```python
from build123d import *
from build123d.topology import SkipClean

# Parameters (mm, degrees)
SKETCH_1_W          = 63
SKETCH_1_H          = 15
SKETCH_1_R          = 1.5
SKETCH_1_R_2        = 1.1
SKETCH_1_R_3        = 2.6
EXTRUDE_1_DEPTH     = 2
SKETCH_2_R          = 1.4
EXTRUDE_2_DEPTH     = 2
SKETCH_3_R          = 3
CUT_EXTRUDE_1_DEPTH = 1.5
SKETCH_4_W          = 46
SKETCH_4_H          = 1.5
EXTRUDE_3_DEPTH     = 5
SKETCH_2_3_R        = 0.95
CUT_EXTRUDE_2_DEPTH = 1.5
CUT_EXTRUDE_3_DEPTH = 0.25
SKETCH_1_7_W        = 15
SKETCH_1_7_H        = 15
SKETCH_1_7_R        = 1.5
SKETCH_1_7_R_2      = 1.1
EXTRUDE_4_DEPTH     = 4
SKETCH_1_8_R        = 6
SKETCH_1_8_R_2      = 1.5
SKETCH_1_8_R_3      = 1.1
CUT_EXTRUDE_4_DEPTH = 2
CUT_EXTRUDE_5_DEPTH = 15
EXTRUDE_START       = 3
SKETCH_8_R          = 5.5
SKETCH_8_R_2        = 2.6
EXTRUDE_11_DEPTH    = 3
CUT_EXTRUDE_6_DEPTH = 3.5
CUT_EXTRUDE_7_DEPTH = 3
SKETCH_8_2_R        = 5.5
SKETCH_8_2_R_2      = 2.6
EXTRUDE_12_DEPTH    = 4


with BuildPart() as part:
    # 草图1 → 凸台-拉伸1 (new body)
    with BuildSketch(Plane(origin=(0, 0, 0), x_dir=(1, 0, 0), z_dir=(0, 1, 0))):
        Rectangle(SKETCH_1_W, SKETCH_1_H)
        with Locations(Location((-8.5, 0, 0), (0, 0, 270))):
            Circle(SKETCH_1_R, mode=Mode.SUBTRACT)
        with Locations(Location((-4.169872981, 2.5, 0), (0, 0, 270))):
            Circle(SKETCH_1_R_2, mode=Mode.SUBTRACT)
        with Locations(Location((-12.830127019, -2.5, 0), (0, 0, 270))):
            Circle(SKETCH_1_R_2, mode=Mode.SUBTRACT)
        with Locations(Location((8, 0, 0), (0, 0, 270))):
            Circle(SKETCH_1_R_3, mode=Mode.SUBTRACT)
        with Locations(Location((24, 0, 0), (0, 0, 270))):
            Circle(SKETCH_1_R, mode=Mode.SUBTRACT)
        with Locations(Location((27.5, 0, 0), (0, 0, 270))):
            Circle(SKETCH_1_R_2, mode=Mode.SUBTRACT)
        with Locations(Location((24, -3.5, 0), (0, 0, 270))):
            Circle(SKETCH_1_R_2, mode=Mode.SUBTRACT)
        with Locations(Location((20.5, 0, 0), (0, 0, 270))):
            Circle(SKETCH_1_R_2, mode=Mode.SUBTRACT)
        with Locations(Location((24, 3.5, 0), (0, 0, 270))):
            Circle(SKETCH_1_R_2, mode=Mode.SUBTRACT)
    extrude(amount=EXTRUDE_1_DEPTH)

    # 草图2 → 凸台-拉伸2 (add)
    with BuildSketch(Plane.XY.offset(7.5)):
        with Locations(Location((-23.5, 0.6, 0), (0, 0, 205.376933525))):
            Circle(SKETCH_2_R)
        with Locations(Location((-8.5, 0.6, 0), (0, 0, 205.376933525))):
            Circle(SKETCH_2_R)
        with Locations(Location((6.5, 0.6, 0), (0, 0, 205.376933525))):
            Circle(SKETCH_2_R)
    extrude(amount=EXTRUDE_2_DEPTH)

    # 草图3 → 切除-拉伸1 (cut)
    with BuildSketch(Plane.XZ):
        with Locations(Location((-8.5, 0, 0), (0, 0, 270))):
            Circle(SKETCH_3_R)
    extrude(amount=-CUT_EXTRUDE_1_DEPTH, mode=Mode.SUBTRACT)

    # 草图4 → 凸台-拉伸3 (add)
    with BuildSketch(Plane.XZ):
        with Locations((-8.5, 6.75)):
            Rectangle(SKETCH_4_W, SKETCH_4_H)
    extrude(amount=EXTRUDE_3_DEPTH)

    # 草图2<3> → 切除-拉伸2 (cut)
    with BuildSketch(Plane.XY.offset(7.5)):
        with Locations((-23.5, -3.4)):
            Circle(SKETCH_2_3_R)
        with Locations((-8.5, -3.4)):
            Circle(SKETCH_2_3_R)
        with Locations((6.5, -3.4)):
            Circle(SKETCH_2_3_R)
    extrude(amount=-CUT_EXTRUDE_2_DEPTH, mode=Mode.SUBTRACT)

    # 草图5 → 切除-拉伸3 (cut)
    with BuildSketch(Plane(origin=(0, 0, 6), x_dir=(-1, 0, 0), z_dir=(0, 0, -1))):
        Polygon((22.403034489, -1.5), (24.596965511, -1.5), (25.693931023, -3.4), (24.596965511, -5.3), (22.403034489, -5.3), (21.306068977, -3.4), align=None)
        Polygon((6.306068977, -3.4), (7.403034489, -1.5), (9.596965511, -1.5), (10.693931023, -3.4), (9.596965511, -5.3), (7.403034489, -5.3), align=None)
        Polygon((-8.693931023, -3.4), (-7.596965511, -1.5), (-5.403034489, -1.5), (-4.306068977, -3.4), (-5.403034489, -5.3), (-7.596965511, -5.3), align=None)
    extrude(amount=-CUT_EXTRUDE_3_DEPTH, mode=Mode.SUBTRACT)

    # 草图1<7> → 凸台-拉伸4 (add)
    with SkipClean():  # the faces are left unmerged after this step: merging them gives an invalid solid
        with BuildSketch(Plane(origin=(0, 0, 0), x_dir=(1, 0, 0), z_dir=(0, 1, 0))):
            with Locations((24, 0)):
                Rectangle(SKETCH_1_7_W, SKETCH_1_7_H)
            with Locations(Location((24, 0, 0), (0, 0, 270))):
                Circle(SKETCH_1_7_R, mode=Mode.SUBTRACT)
            with Locations(Location((27.5, 0, 0), (0, 0, 270))):
                Circle(SKETCH_1_7_R_2, mode=Mode.SUBTRACT)
            with Locations(Location((24, -3.5, 0), (0, 0, 270))):
                Circle(SKETCH_1_7_R_2, mode=Mode.SUBTRACT)
            with Locations(Location((20.5, 0, 0), (0, 0, 270))):
                Circle(SKETCH_1_7_R_2, mode=Mode.SUBTRACT)
            with Locations(Location((24, 3.5, 0), (0, 0, 270))):
                Circle(SKETCH_1_7_R_2, mode=Mode.SUBTRACT)
        extrude(amount=EXTRUDE_4_DEPTH)

    # 草图1<8> → 切除-拉伸4 (cut)
    with SkipClean():  # the faces are left unmerged after this step: merging them gives an invalid solid
        with BuildSketch(Plane(origin=(0, 0, 0), x_dir=(1, 0, 0), z_dir=(0, 1, 0))):
            with Locations(Location((24, 0, 0), (0, 0, 270))):
                Circle(SKETCH_1_8_R)
            with Locations(Location((24, 0, 0), (0, 0, 270))):
                Circle(SKETCH_1_8_R_2, mode=Mode.SUBTRACT)
            with Locations(Location((27.5, 0, 0), (0, 0, 270))):
                Circle(SKETCH_1_8_R_3, mode=Mode.SUBTRACT)
            with Locations(Location((24, -3.5, 0), (0, 0, 270))):
                Circle(SKETCH_1_8_R_3, mode=Mode.SUBTRACT)
            with Locations(Location((20.5, 0, 0), (0, 0, 270))):
                Circle(SKETCH_1_8_R_3, mode=Mode.SUBTRACT)
            with Locations(Location((24, 3.5, 0), (0, 0, 270))):
                Circle(SKETCH_1_8_R_3, mode=Mode.SUBTRACT)
        extrude(amount=CUT_EXTRUDE_4_DEPTH, mode=Mode.SUBTRACT)

    # 草图6 → 切除-拉伸5 (cut)
    with BuildSketch(Plane(origin=(0, 0, -7.5), x_dir=(-1, 0, 0), z_dir=(0, 0, -1))):
        Polygon((-16.5, 2), (-18.5, 4), (-16.5, 4), align=None)
    extrude(amount=-CUT_EXTRUDE_5_DEPTH, mode=Mode.SUBTRACT)

    # 草图8 → 凸台-拉伸11 (add)
    with SkipClean():  # the faces are left unmerged after this step: merging them gives an invalid solid
        with BuildSketch(Plane.XZ.offset(EXTRUDE_START)):
            with Locations(Location((8, 0, 0), (0, 0, 90))):
                Circle(SKETCH_8_R)
            with Locations(Location((8, 0, 0), (0, 0, 270))):
                Circle(SKETCH_8_R_2, mode=Mode.SUBTRACT)
        extrude(amount=-EXTRUDE_11_DEPTH)

    # 草图10 → 切除-拉伸6 (cut)
    with BuildSketch(Plane.XZ.offset(3)):
        Polygon((8, 3.175426481), (5.25, 1.58771324), (5.25, -1.58771324), (8, -3.175426481), (10.75, -1.58771324), (10.75, 1.58771324), align=None)
    extrude(amount=-CUT_EXTRUDE_6_DEPTH, mode=Mode.SUBTRACT)

    # 草图11 → 切除-拉伸7 (cut)
    with BuildSketch(Plane.XZ.offset(3)):
        with BuildLine():
            Line((3.101020514, 2.5), (12.898979486, 2.5))
            ThreePointArc((12.898979486, 2.5), (8, 5.5), (3.101020514, 2.5))
        make_face()
    extrude(amount=-CUT_EXTRUDE_7_DEPTH, mode=Mode.SUBTRACT)

    # 草图8<2> → 凸台-拉伸12 (add)
    with BuildSketch(Plane.XZ):
        with Locations(Location((8, 0, 0), (0, 0, 270))):
            Circle(SKETCH_8_2_R)
        with Locations(Location((8, 0, 0), (0, 0, 270))):
            Circle(SKETCH_8_2_R_2, mode=Mode.SUBTRACT)
    extrude(amount=-EXTRUDE_12_DEPTH)


solid = part.part
```
Verification items for the finished model (mm, model axes). A direction names the side the tool comes from. Give positions to 0.01 mm unless a question says otherwise; leave off trailing zeros. Order: outer loops, then holes, each group sorted by start corner. A loop starts at its lowest first (then second) coordinate and runs counter-clockwise, first axis right, second up. Notation, with made-up numbers: (20, 81) -> (60, 81) arc R13 cw to (60, 106) -> close; hole circle Ø3 at (-8, 30). An arc over 180 degrees is marked (long way). One line per item, written item: value.
(1) Draft check along Y on faces 1 (the face through (5.8, -2.76, 6.88)), 2 (the face through (26, 4, 0)), 3 (the face through (-24.9, 0.53, 8.49)), 4 (the face through (5.25, -2, 0)). Enter one of: pulls with the +Y half, pulls with the -Y half, needs draft (parallel to the pull), parting line crosses it, or undercut.
Final values:
face 1: undercut
face 2: pulls with the +Y half
face 3: parting line crosses it
face 4: needs draft
(2) Sectioned sample at C-C on y = 0.6. Record the cut outline in (x, z).
Final values:
outline: (-31.5, -7.5) -> (31.5, -7.5) -> (31.5, 7.5) -> (7.9, 7.5) -> (7.9, 9.5) -> (5.1, 9.5) -> (5.1, 7.5) -> (-7.1, 7.5) -> (-7.1, 9.5) -> (-9.9, 9.5) -> (-9.9, 7.5) -> (-22.1, 7.5) -> (-22.1, 9.5) -> (-24.9, 9.5) -> (-24.9, 7.5) -> (-31.5, 7.5) -> close; hole circle Ø2.2 at (-12.83, 2.5); hole circle Ø6 at (-8.5, 0); hole circle Ø2.2 at (-4.17, -2.5); hole circle Ø5.2 at (8, 0); hole circle Ø12 at (24, 0)
(3) Sectioned sample at A-A on x = 27.5. Record the cut outline in (y, z).
Final values:
outline: (0, -7.5) -> (4, -7.5) -> (4, -1.1) -> (2, -1.1) -> (2, -4.87) -> (0, -4.87) -> close; (0, 4.87) -> (2, 4.87) -> (2, 1.1) -> (4, 1.1) -> (4, 7.5) -> (0, 7.5) -> close
(4) Sectioned sample at B-B on z = 0. Count the separate pieces of the cut face and the enclosed holes in it, then the cut area to 3 significant figures.
Final values:
separate pieces: 6
enclosed holes: 0
area: 122 mm^2
(5) Scan lines: line 1 along X through (y, z) = (1.15, 0); line 2 along X through (y, z) = (2.75, 1.75); line 3 along X through (y, z) = (3.65, 0). Record each from-to range of solid material in increasing order. Write a range as [from, to].
Final values:
line 1: [-31.5, -11.5], [-5.5, 5.4], [10.6, 18], [30, 31.5]
line 2: [2.79, 6.08], [9.92, 13.21], [17.25, 31.5]
line 3: [2.5, 5.4], [10.6, 13.5], [18.15, 19.4], [21.6, 22.5], [25.5, 26.4], [28.6, 31.5]
(6) Gauge pin test, flat ends, axial feed: pin 1 (2.5 mm diameter, centred on y = -1.5, z = 0, fed in from -X); pin 2 (3 mm diameter, centred on x = 6.5, y = -3.4, fed in from -Z); pin 3 (4 mm diameter, centred on x = 9, z = -0.5, fed in from -Y). Record the tip position at first contact, or that the pin passes through.
Final values:
pin 1: x = 2.5
pin 2: z = -5.5
pin 3: y = -3
(7) Tool access check on faces 5 (the face through (6, -2, 6.25)), 6 (the face through (5.46, 1.97, 0.56)), 7 (the face through (-5.526, 0.74, 0.391)). Record the directions out of +Z, -Z, +X, -X, +Y, -Y that give a thin tool (end or side, any length) a straight path to the whole face; none if there is none.
Final values:
face 5: none
face 6: +Y, -Y
face 7: -Y
